Print and shaded views of the part. All mm, measured from the part's lowest x, y and z. A direction names the side the tool comes from. Round coordinates to 2 decimals unless told otherwise and drop trailing zeros. Loops run counter-clockwise (first coordinate to the right, second up) from the corner with the lowest first, then second, coordinate; pieces in that order, holes last. Notation, with made-up numbers: (18.25, -21.75) -> (77.25, -21.75) arc R16 ccw to (77.25, 6.25) -> close; hole circle Ø10 at (77.5, -36.5). An arc over 180 degrees is marked (long way). Answer as CSV lines item,"result".
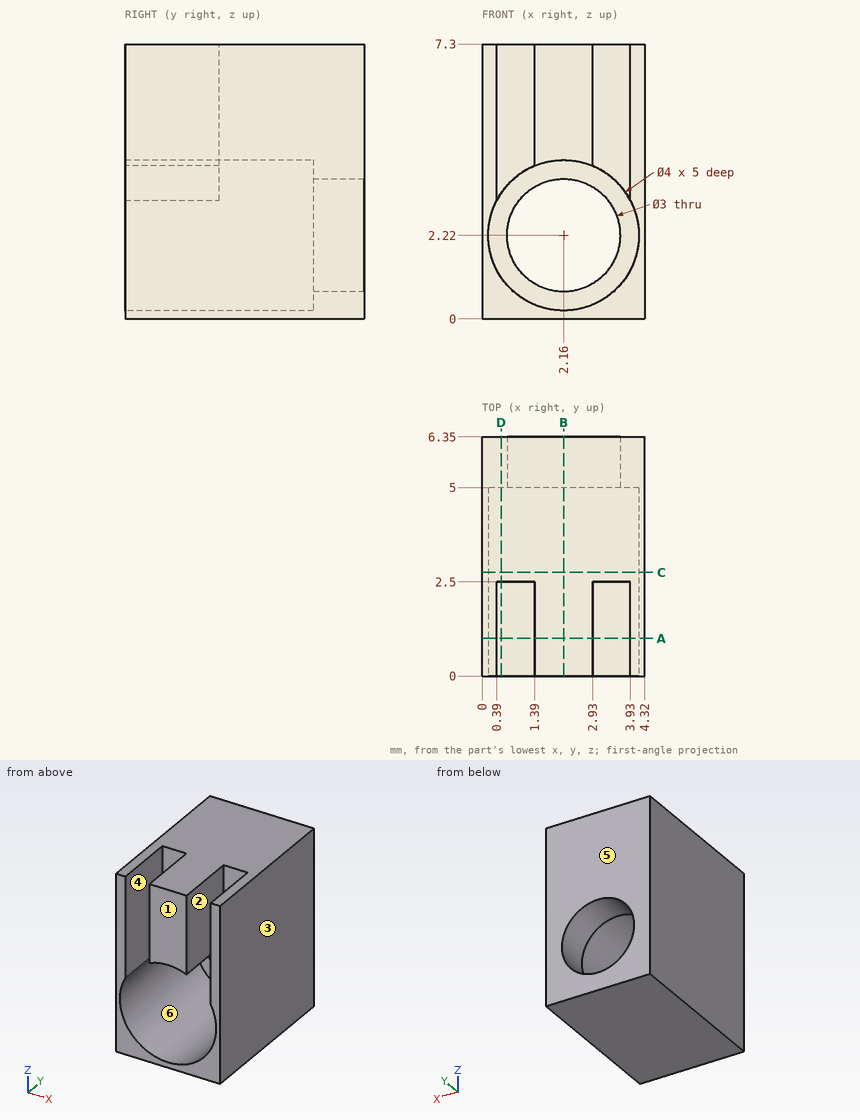
Q1. Slice it at A-A, the plane y = 1. Give the cut face in (x, z).
Results:
outline,"(0, 0) -> (4.32, 0) -> (4.32, 7.3) -> (3.93, 7.3) -> (3.93, 3.15) arc R2 cw (long way) to (0.39, 3.15) -> (0.39, 7.3) -> (0, 7.3) -> close; (1.39, 4.07) arc R2 cw to (2.93, 4.07) -> (2.93, 7.3) -> (1.39, 7.3) -> close"
Q2. Slice it at B-B, the plane x = 2.16. Give the cut face in (y, z).
Results:
outline,"(0, 0) -> (6.35, 0) -> (6.35, 0.72) -> (5, 0.72) -> (5, 0.22) -> (0, 0.22) -> close; (0, 4.22) -> (5, 4.22) -> (5, 3.72) -> (6.35, 3.72) -> (6.35, 7.3) -> (0, 7.3) -> close"
Q3. Drop flat-ended pins along their axis: pin 1 Ø1.2 at (x, z) = (3, 1.5) entering from -Y; pin 2 Ø2.5 at (x, z) = (2.16, 2.22) entering from +Y. Give the stop position or say it passes through.
Results:
pin 1,"y = 5"
pin 2,"through"
Q4. Tool access for the marked faces 4, 5 and 6: list every direction of +Z, -Z, +X, -X, +Y, -Y with a clear straight run to the whole face (end or side of a thin tool).
Results:
face 4,"+Z, -Y"
face 5,"+Z, -Z, +X, -X, +Y"
face 6,"-Y"
Q5. Probe L1, parallel to X at y = 1.25, z = 2.22; L2, parallel to X at y = 5.75, z = 2.22; L3, parallel to X at y = 0.75, z = 6. List the from-to ranges inside material, lowest first. Write a range as [from, to].
Results:
L1,"[0, 0.16], [4.16, 4.32]"
L2,"[0, 0.66], [3.66, 4.32]"
L3,"[0, 0.39], [1.39, 2.93], [3.93, 4.32]"
Q6. Two-plate mould, pull along X, no slides. Class the marked faces 1, 2 and 3: pulls with the +X half, pulls with the -X half, needs draft (parallel to the pull), parting line crosses it, or undercut.
Results:
face 1,"needs draft"
face 2,"undercut"
face 3,"pulls with the +X half"
Q7. Slice it at C-C, the plane y = 2.75. Give the cut face in (x, z), and give its area (3 significant figures).
Results:
outline,"(0, 0) -> (4.32, 0) -> (4.32, 7.3) -> (0, 7.3) -> close; hole circle Ø4 at (2.16, 2.22)"
area,"19.0 mm2"
Q8. Slice it at D-D, the plane x = 0.5. Give the cut face in (y, z).
Results:
outline,"(0, 0) -> (6.35, 0) -> (6.35, 7.3) -> (2.5, 7.3) -> (2.5, 3.34) -> (5, 3.34) -> (5, 1.1) -> (0, 1.1) -> close"
